Geometry: final body of the model. Coordinates: model frame, mm. Give positions to 0.01 mm unless a question says otherwise; leave off trailing zeros. Order: outer loops, then holes, each group sorted by start corner. A loop starts at its lowest first (then second) coordinate and runs counter-clockwise, first axis right, second up. Notation, with made-up numbers: (1.5, -2) -> (40.5, -2) arc R24 cw to (40.5, 27) -> close; hole circle Ø9 at (50.5, 49.5). An arc over 180 degrees is marked (long way). Answer in a Markdown table with one row per item. Add a question column.
Q1. Contact query for flat-ended pins moving along their axis: P1, Ø11.5, axis at y = -25.4, z = 0, coming from the +X side; P2, Ø4, axis at y = -98, z = 7, coming from the +X side; P3, Ø1, axis at y = -78, z = -4.5, coming from the -X side; P4, Ø1, axis at x = 3, y = -21, coming from the +Z side. Output: stop coordinate, or through.
Q2. Cut plane C-C on y = -25.4. Return the cut outline in (x, z) (3 decimals), and give its area (3 significant figures).
Q3. Line query: line 1 along Y through (x, z) = (8.5, 0); line 2 along Z through (x, y) = (11.5, -25.4); line 3 along Y through (x, z) = (-10.5, -3.5). Output: solid intervals per line, ascending. Write a range as from..to.
Q4. Cut plane B-B on y = -142. Return the cut outline in (x, z) (3 decimals).
Q5. Cut plane A-A on z = 0. Return the cut outline in (x, y) (3 decimals), and give its area (3 significant figures).
from build123d import *

# Parameters (mm, degrees)
F0_R     = 15.875
F1_DEPTH = 171.45
F2_R     = 6.35
F3_DEPTH = 25.4
F4_DEPTH = 25.4
F5_SIZE2 = 3.048
F5_SIZE  = 1.27
F6_SIZE2 = 3.048
F6_SIZE  = 1.27


with BuildPart() as f1:
    # F0 (on Front) → F1 (new body)
    with BuildSketch(Plane.XZ):
        Circle(F0_R)
    extrude(amount=F1_DEPTH)

    # F2 (on Right) → F3 (cut)
    with BuildSketch(Plane.YZ):
        with Locations((-25.4, 0)):
            Circle(F2_R)
    extrude(amount=-F3_DEPTH, mode=Mode.SUBTRACT)

    # F4 (cut): a face of the model
    f4_faces = [f1.faces().sort_by_distance(p)[0] for p in [
        (0, -25.4, 0),
    ]]
    extrude(f4_faces, amount=-F4_DEPTH, mode=Mode.SUBTRACT)

    # F5
    f5_edges = [f1.edges().sort_by_distance(p)[0] for p in [
        (-15.875, -171.45, 0),
    ]]
    f5_side = f1.faces().sort_by_distance((0, -171.45, 0))[0]
    chamfer(f5_edges, length=F5_SIZE, length2=F5_SIZE2, reference=f5_side)

    # F6
    f6_edges = [f1.edges().sort_by_distance(p)[0] for p in [
        (-15.875, 0, 0),
    ]]
    f6_side = f1.faces().sort_by_distance((0, 0, 0))[0]
    chamfer(f6_edges, length=F6_SIZE, length2=F6_SIZE2, reference=f6_side)


solid = f1.part
Completed:
| question | item | result |
|---|---|---|
| 1 | P1 | passes through |
| 1 | P2 | stops at x = 15.07 |
| 1 | P3 | stops at x = -15.36 |
| 1 | P4 | stops at z = 15.68 |
| 2 | outline | (-14.55, -6.35) arc R15.875 ccw to (14.55, -6.35) -> close; (-14.55, 6.35) -> (14.55, 6.35) arc R15.875 ccw to start |
| 2 | area | 400 mm² |
| 3 | line 1 | y = -171.45..-31.75, -19.05..0 |
| 3 | line 2 | z = -10.94..-6.35, 6.35..10.94 |
| 3 | line 3 | y = -171.45..-30.7, -20.1..0 |
| 4 | outline | circle Ø31.75 at (0, 0) |
| 5 | outline | (-15.875, -168.402) -> (-14.605, -171.45) -> (14.605, -171.45) -> (15.875, -168.402) -> (15.875, -31.75) -> (-15.875, -31.75) -> close; (-15.875, -19.05) -> (15.875, -19.05) -> (15.875, -3.048) -> (14.605, 0) -> (-14.605, 0) -> (-15.875, -3.048) -> close |
| 5 | area | 5,030 mm² |
